Work out the finished part from the listing and answer in its coordinate system (mm). Face numbers are marked on the shaded views. Coordinates: 2 decimals unless noted, no trailing zeros. Loops run counter-clockwise (first coordinate to the right, second up) from the corner with the lowest first, then second, coordinate; pieces in that order, holes last. Notation, with made-up numbers: (27, -9.75) -> (50, -9.75) arc R21 ccw to (50, 20.25) -> close; hole circle Ø10 at (-29, 55.25). An arc over 180 degrees is marked (long way). Use a Markdown table: item, result.
Autodesk Inventor part; units mm, degrees
ref_plane "YZ Plane" through (0, 0, 0) normal (1, 0, 0) x (0, 1, 0)
ref_plane "XZ Plane" through (0, 0, 0) normal (0, 1, 0) x (-1, 0, 0)
ref_plane "XY Plane" through (0, 0, 0) normal (0, 0, 1) x (1, 0, 0)
sketch "Sketch1" plane through (0, 0, 0) normal (0, 1, 0) x (-1, 0, 0)
  point P0 (0, 0)
sketch "Sketch2" plane through (0, 0, 0) normal (0, 1, 0) x (-1, 0, 0)
  line L0 (0, 0) -> (150, 0)
  line L1 (150, 0) -> (150, -150)
  line L2 (150, -150) -> (0, -150)
  line L3 (0, -150) -> (0, 0)
  dimension "d0" = 150
  dimension "d1" = 150
extrude "Extrusion1" add sketch "Sketch2" along normal blind 7.5
sketch "Sketch4" plane through (0, 7.5, 0) normal (0, 1, 0) x (1, 0, 0)
  line L0 (0, 0) -> (-150, 0)
  line L1 (0, 150) -> (0, 0)
  line L2 (-150, 0) -> (0, 0)
  line L3 (0, 0) -> (0, 150)
  line L4 (0, 150) -> (-150, 150)
  line L5 (-150, 150) -> (-150, 0)
  line L6 (-146, 4) -> (-4, 4)
  line L7 (-4, 4) -> (-4, 146)
  line L8 (-4, 146) -> (-146, 146)
  line L9 (-146, 146) -> (-146, 4)
  dimension "d7" = 4
extrude "Extrusion3" add sketch "Sketch4" along normal blind 35
sketch "Sketch5" plane through (0, 7.5, 0) normal (0, 1, 0) x (1, 0, 0)
  line L0 (-146, 146) -> (-146, 4)
  line L1 (-146, 4) -> (-136, 4)
  line L2 (-136, 4) -> (-136, 14)
  line L3 (-136, 14) -> (-146, 14)
  line L4 (-146, 14) -> (-146, 4)
  point P0 (0, 0)
  dimension "d10" = 10
  dimension "d11" = 10
extrude "Extrusion4" add sketch "Sketch5" along normal blind 35
pattern_linear "Rectangular Pattern1" count 2 spacing 132 along (0, 0, -1) count 2 spacing 132 along (1, 0, 0) of "Extrusion4"
sketch "Sketch6" plane through (0, 42.5, 0) normal (0, 1, 0) x (1, 0, 0)
  line L0 (-136, 14) -> (-146, 14)
  line L1 (-141, 14) -> (-141, 0)
  line L2 (0, 0) -> (-150, 0)
  circle A0 centre (-141, 9) radius 2.75
  dimension "d20" = 5.5
extrude "Extrusion5" cut sketch "Sketch6" against normal blind 80
pattern_linear "Rectangular Pattern2" count 2 spacing 132 along (0, 0, -1) count 2 spacing 132 along (1, 0, 0) of "Extrusion5"
sketch "Sketch9" plane through (0, 42.5, 0) normal (0, 1, 0) x (1, 0, 0)
  point P0 (0, 0)
sketch "Sketch10" plane through (0, 42.5, 0) normal (0, 1, 0) x (1, 0, 0)
  line L0 (0, 0) -> (-150, 0)
  line L1 (-150, 150) -> (-150, 0)
  line L2 (0, 0) -> (-150, 0)
  line L3 (-150, 0) -> (-150, 150)
  line L4 (-150, 150) -> (0, 150)
  line L5 (0, 150) -> (0, 0)
  line L6 (-136, 4) -> (-14, 4)
  line L7 (-14, 4) -> (-136, 4)
  line L8 (-136, 4) -> (-136, 14)
  line L9 (-136, 4) -> (-136, 14)
  line L10 (-146, 14) -> (-136, 14)
  line L11 (-136, 14) -> (-146, 14)
  line L12 (-146, 136) -> (-146, 14)
  line L13 (-146, 14) -> (-146, 136)
  line L14 (-146, 136) -> (-136, 136)
  line L15 (-14, 146) -> (-136, 146)
  line L16 (-136, 136) -> (-136, 146)
  line L17 (-14, 136) -> (-14, 146)
  line L18 (-136, 146) -> (-14, 146)
  line L19 (-14, 146) -> (-14, 136)
  line L20 (-4, 136) -> (-14, 136)
  line L21 (-14, 136) -> (-4, 136)
  line L22 (-4, 136) -> (-4, 14)
  line L23 (-4, 14) -> (-14, 14)
  line L24 (-4, 14) -> (-14, 14)
  line L25 (-14, 14) -> (-14, 4)
  line L26 (-14, 14) -> (-14, 4)
  circle A0 centre (-9, 9) radius 2.75
  circle A1 centre (-141, 9) radius 2.75
  circle A2 centre (-141, 141) radius 2.75
  circle A3 centre (-141, 141) radius 2.75
  circle A4 centre (-9, 141) radius 2.75
  circle A5 centre (-9, 141) radius 2.75
extrude "Extrusion8" add sketch "Sketch10" along normal blind 70
sketch "Sketch11" plane through (0, 0, -150) normal (0, 0, -1) x (-1, 0, 0)
  point P0 (0, 0)
sketch "Sketch12" plane through (0, 0, -150) normal (0, 0, -1) x (-1, 0, 0)
  circle A0 centre (29.7835, 83.8626) radius 3.25
  point P0 (0, 0)
  dimension "d47" = 6.5
extrude "Extrusion9" cut sketch "Sketch12" against normal blind 70
pattern_linear "Rectangular Pattern5" count 3 spacing 10 along (-1, 0, 0) of "Extrusion9"
sketch "Sketch13" plane through (0, 0, -150) normal (0, 0, -1) x (-1, 0, 0)
  line L0 (26.5335, 75.8795) -> (106.5335, 75.8795)
  line L1 (106.5335, 75.8795) -> (106.5335, 68.3795)
  line L2 (106.5335, 68.3795) -> (26.5335, 68.3795)
  line L3 (26.5335, 68.3795) -> (26.5335, 75.8795)
  point P0 (0, 0)
  dimension "d53" = 80
  dimension "d54" = 7.5
extrude "Extrusion10" cut sketch "Sketch13" against normal blind 70
sketch "Sketch14" plane through (-136, 7.5, -146) normal (0, 0, 1) x (1, 0, 0)
  point P0 (136, -7.5)
sketch "Sketch15" plane through (-136, 7.5, -146) normal (0, 0, 1) x (1, 0, 0)
  point P0 (136, -7.5)
sketch "Sketch16" plane through (0, 0, -150) normal (0, 0, -1) x (-1, 0, 0)
  circle A0 centre (29.7835, 51.6304) radius 6.25
  point P0 (0, 0)
  dimension "d57" = 12.5
extrude "Extrusion11" cut sketch "Sketch16" against normal blind 70
properties part number "Bottom"
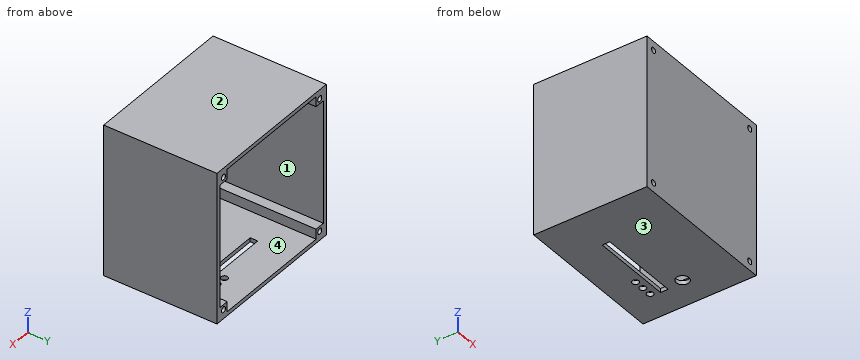
Q1. Given pin 1 Ø2 at (x, z) = (-133, -80.5) entering from +Y; pin 2 Ø3.5 at (x, z) = (-141, -9) entering from -Y, each flat-ended and moving along its own axis, determine where each tip first touches the part or whether it passes through.
Solved:
| item | result |
|---|---|
| pin 1 | y = 7.5 |
| pin 2 | through |
Q2. Section B-B on y = 23 is taken. Determine the outline of the cut face in (x, z), and give its area (3 significant figures).
Solved:
| item | result |
|---|---|
| outline | (-150, -150) -> (0, -150) -> (0, 0) -> (-150, 0) -> close; hole (-146, -136) -> (-136, -136) -> (-136, -146) -> (-14, -146) -> (-14, -136) -> (-4, -136) -> (-4, -14) -> (-14, -14) -> (-14, -4) -> (-136, -4) -> (-136, -14) -> (-146, -14) -> close; hole circle Ø5.5 at (-141, -141); hole circle Ø5.5 at (-141, -9); hole circle Ø5.5 at (-9, -141); hole circle Ø5.5 at (-9, -9) |
| area | 2,640 mm² |
Q3. Section D-D on x = -100 is taken. Determine the outline of the cut face in (y, z).
Solved:
| item | result |
|---|---|
| outline | (0, -150) -> (68.38, -150) -> (68.38, -146) -> (7.5, -146) -> (7.5, -4) -> (112.5, -4) -> (112.5, 0) -> (0, 0) -> close; (75.88, -150) -> (112.5, -150) -> (112.5, -146) -> (75.88, -146) -> close |
Q4. Consider line 1 (Z direction, x = -141, y = 25.5); line 2 (Z direction, x = -48.5, y = 45.5). Determine where each line is inside the solid, lowest interval first. Write a range as [from, to].
Solved:
| item | result |
|---|---|
| line 1 | [-150, -143.75], [-138.25, -136], [-14, -11.75], [-6.25, 0] |
| line 2 | [-150, -146], [-4, 0] |
Q5. Determine the mould class of the marked faces 1, 2, 3 and 4 for opening direction Z: pulls with the +Z half, pulls with the -Z half, needs draft (parallel to the pull), parting line crosses it, or undercut.
Solved:
| item | result |
|---|---|
| face 1 | undercut |
| face 2 | pulls with the +Z half |
| face 3 | pulls with the -Z half |
| face 4 | undercut |
Q6. Section A-A on x = -141 is taken. Determine the outline of the cut face in (y, z).
Solved:
| item | result |
|---|---|
| outline | (0, -150) -> (112.5, -150) -> (112.5, -143.75) -> (0, -143.75) -> close; (0, -138.25) -> (112.5, -138.25) -> (112.5, -136) -> (7.5, -136) -> (7.5, -14) -> (112.5, -14) -> (112.5, -11.75) -> (0, -11.75) -> close; (0, -6.25) -> (112.5, -6.25) -> (112.5, 0) -> (0, 0) -> close |
Q7. Section C-C on z = -141 is taken. Determine the outline of the cut face in (x, y), and give its area (3 significant figures).
Solved:
| item | result |
|---|---|
| outline | (-150, 0) -> (-143.75, 0) -> (-143.75, 112.5) -> (-150, 112.5) -> close; (-138.25, 0) -> (-11.75, 0) -> (-11.75, 112.5) -> (-14, 112.5) -> (-14, 7.5) -> (-136, 7.5) -> (-136, 112.5) -> (-138.25, 112.5) -> close; (-6.25, 0) -> (0, 0) -> (0, 112.5) -> (-6.25, 112.5) -> close |
| area | 2,830 mm² |
